Check sheet for the modelled part. Datum: model origin and axes. Units: mm. Face numbers are marked on the shaded views. A direction names the side the tool comes from. Give positions to 0.01 mm unless a question says otherwise; leave off trailing zeros. Loops run counter-clockwise (first coordinate to the right, second up) from the corner with the lowest first, then second, coordinate; pieces in that order, holes last. Notation, with made-up numbers: (42, 18) -> (73, 18) arc R37 ccw to (73, 54) -> close; hole circle Ø9 at (-33, 25.5). An arc over 180 degrees is marked (long way). Answer as CSV lines item,"result". Start each with the question number.
(1) Section check C-C on z = 14. Enter the section's corners in (x, y).
(2) Material ranges on line 1 (Z direction, x = -2.75, y = -1); line 2 (Y direction, x = -0.25, z = 44); line 3 (X direction, y = 1, z = 29), recorded low to high. Write a range as from..to.
(3) Section check A-A on x = 0. Enter the section's corners in (y, z).
(4) Section check B-B on y = 0. Enter the section's corners in (x, z), plus the area to 3 significant figures.
(5) Section check D-D on z = 32.5. Enter the section's corners in (x, y), plus the area to 3 significant figures.
(6) Gauge pin test, flat ends, axial feed: pin 1 Ø1.5 at (x, z) = (2, 47.5) entering from -Y; pin 2 Ø0.6 at (y, z) = (0, 29) entering from +X; pin 3 Ø1.5 at (x, z) = (2, 31) entering from +Y. Record the tip position at first contact, or that the pin passes through.
(7) Access from +Z, -Z, +X, -X, +Y, -Y to the whole of each face (thin tool, end or side, straight path). Record for the marked faces 1, 2, 3 and 4.
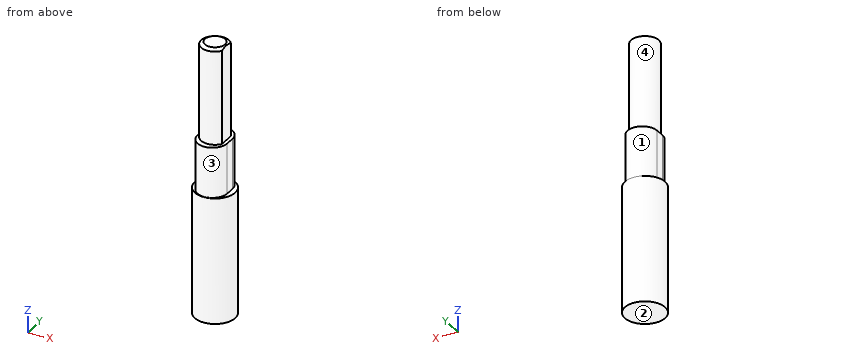
from build123d import *

# Parameters (mm, degrees)
F0_R     = 4
F1_DEPTH = 25
F3_DEPTH = 10
F4_R     = 2.75
F5_DEPTH = 19
F6_SIZE2 = 0.4330127019
F6_SIZE  = 0.75
F8_DEPTH = 19


with BuildPart() as f1:
    # F0 (on Top) → F1 (new body)
    with BuildSketch(Plane.XY):
        Circle(F0_R)
    extrude(amount=F1_DEPTH)

    # F2 (on face) → F3 (join)
    with BuildSketch(Plane.XY.offset(25)):
        with BuildLine():
            ThreePointArc((0, -3.9), (2.0859650045, -3.0359650045), (2.95, -0.95))
            Line((2.95, -0.95), (2.95, 0.95))
            ThreePointArc((2.95, 0.95), (2.0859650045, 3.0359650045), (0, 3.9))
            ThreePointArc((0, 3.9), (-2.0859650045, 3.0359650045), (-2.95, 0.95))
            Line((-2.95, 0.95), (-2.95, -0.95))
            ThreePointArc((-2.95, -0.95), (-2.0859650045, -3.0359650045), (0, -3.9))
        make_face()
    extrude(amount=F3_DEPTH)

    # F4 (on face) → F5 (join)
    with BuildSketch(Plane.XY.offset(35)):
        Circle(F4_R)
    extrude(amount=F5_DEPTH)

    # F6
    f6_edges = [f1.edges().sort_by_distance(p)[0] for p in [
        (-2.75, 0, 54),
    ]]
    f6_side = f1.faces().sort_by_distance((0, 0, 54))[0]
    chamfer(f6_edges, length=F6_SIZE, length2=F6_SIZE2, reference=f6_side)

    # F7 (on face) → F8 (cut)
    with BuildSketch(Plane.XY.offset(54)):
        Polygon((2.25, 2.9586648743), (2.25, 0), (2.25, -3.3952166559), (3.5037237976, -3.3952166559), (3.5037237976, 2.9586648743), align=None)
    extrude(amount=-F8_DEPTH, mode=Mode.SUBTRACT)


solid = f1.part
Working result:
1,outline,"circle Ø8 at (0, 0)"
2,line 1,"z = 0..35"
2,line 2,"y = -2.74..2.74"
2,line 3,"x = -2.95..2.95"
3,outline,"(-4, 0) -> (4, 0) -> (4, 25) -> (3.9, 25) -> (3.9, 35) -> (2.75, 35) -> (2.75, 53.57) -> (2, 54) -> (-2, 54) -> (-2.75, 53.57) -> (-2.75, 35) -> (-3.9, 35) -> (-3.9, 25) -> (-4, 25) -> close"
4,outline,"(-4, 0) -> (4, 0) -> (4, 25) -> (2.95, 25) -> (2.95, 35) -> (2.25, 35) -> (2.25, 53.86) -> (2, 54) -> (-2, 54) -> (-2.75, 53.57) -> (-2.75, 35) -> (-2.95, 35) -> (-2.95, 25) -> (-4, 25) -> close"
4,area,"354 mm^2"
5,outline,"(-2.95, -0.95) arc R2.95 ccw to (2.95, -0.95) -> (2.95, 0.95) arc R2.95 ccw to (-2.95, 0.95) -> close"
5,area,"38.5 mm^2"
6,pin 1,"stops at y = -2.45"
6,pin 2,"stops at x = 2.95"
6,pin 3,"stops at y = 3.62"
7,face 1,"+Z, +Y"
7,face 2,"-Z, +X, -X, +Y, -Y"
7,face 3,"+Z, -Y"
7,face 4,"+Z"
